Answer from the drawing. Dimensions are ordinates in mm from the lowest x, y and z of the part. A direction names the side the tool comes from. Coordinates: 2 decimals unless noted, no trailing zeros. Loops run counter-clockwise (first coordinate to the right, second up) from the corner with the lowest first, then second, coordinate; pieces in that order, holes last. Notation, with made-up numbers: (53.25, 66.5) - (107.25, 66.5) arc R24 ccw to (107.25, 86.5) - close; hole circle Ø1 at (42, 42.25). An arc over 180 degrees is marked (long way). Use one line per item in the form item = value. Start each with the question number.
1) A cutting plane is placed at A-A (z = 37). Give the vertices of the cut face in (x, y).
2) Each of these flat-tipped pins is pushed along its axis until it touches: P1, Ø20.5, axis at x = 91, y = 65, coming from the +Z side; P2, Ø6, axis at y = 8, z = 78.5, coming from the -X side; P3, Ø1.5, axis at x = 19, y = 46, coming from the -Z side; P4, Ø12.5, axis at x = 66, y = 62, coming from the +Z side. Where does it stop, or does it pass through?
3) A cutting plane is placed at C-C (z = 68). Give the vertices of the cut face in (x, y).
4) Which of the six approach directions +Z, -Z, +X, -X, +Y, -Y give full straight-line access (tool end or side, diameter ignored) to the marked faces 4, 5 and 6?
5) A cutting plane is placed at D-D (x = 66). Give the vertices of the cut face in (y, z).
6) The mould has two halves that part along X. Classify the marked faces 1, 2 and 3: released by +X, released by -X, zero draft, split by the parting line, or undercut.
7) A cutting plane is placed at B-B (y = 59). Give the vertices of the cut face in (x, z).
8) Consider line 1 (X direction, y = 58, z = 42); line 2 (X direction, y = 4, z = 89); line 3 (Y direction, x = 93.5, z = 17.5). Determine where each line is inside the solid, lowest interval first.
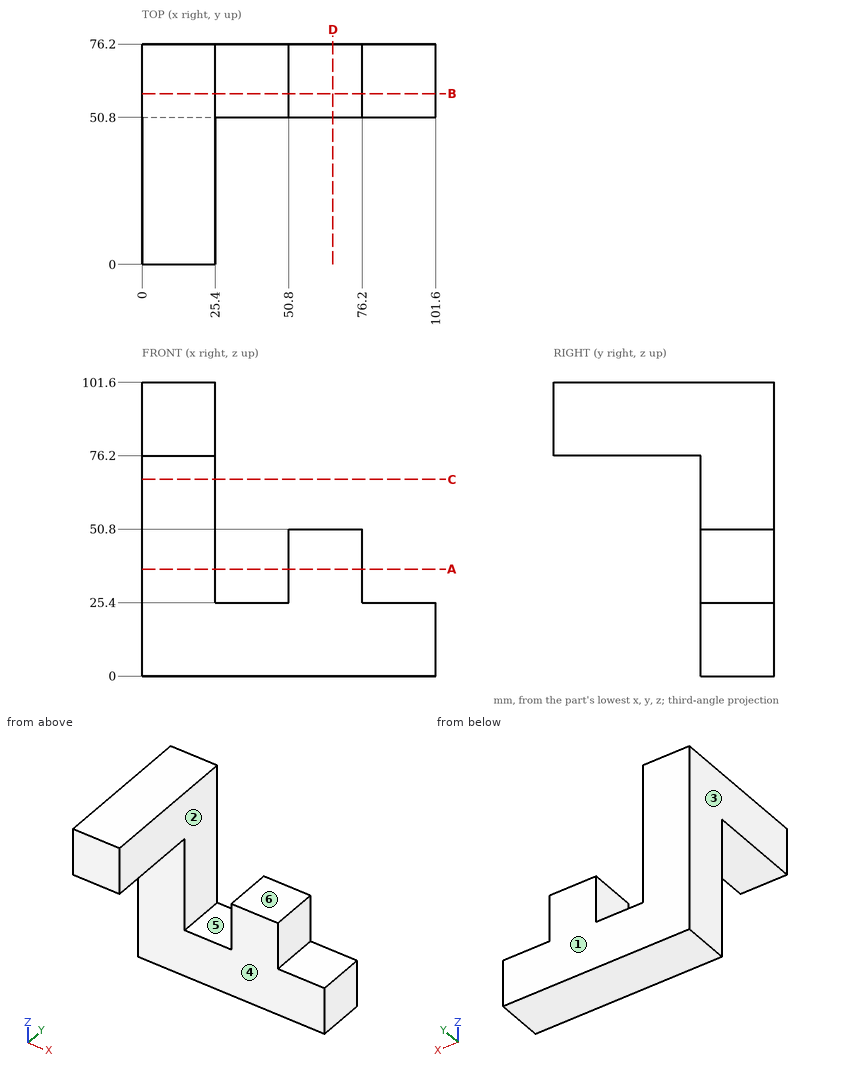
Found:
q1.outline = (0, 50.8) - (25.4, 50.8) - (25.4, 76.2) - (0, 76.2) - close; (50.8, 50.8) - (76.2, 50.8) - (76.2, 76.2) - (50.8, 76.2) - close
q2.P1 = 25.4
q2.P2 = 0
q2.P3 = 76.2
q2.P4 = 50.8
q3.outline = (0, 50.8) - (25.4, 50.8) - (25.4, 76.2) - (0, 76.2) - close
q4.face_4 = -Z, +X, -X, -Y
q4.face_5 = +Z, +Y, -Y
q4.face_6 = +Z, +X, +Y, -Y
q5.outline = (50.8, 0) - (76.2, 0) - (76.2, 50.8) - (50.8, 50.8) - close
q6.face_1 = zero draft
q6.face_2 = undercut
q6.face_3 = released by -X
q7.outline = (0, 0) - (101.6, 0) - (101.6, 25.4) - (76.2, 25.4) - (76.2, 50.8) - (50.8, 50.8) - (50.8, 25.4) - (25.4, 25.4) - (25.4, 101.6) - (0, 101.6) - close
q8.line_1 = 0 to 25.4, 50.8 to 76.2
q8.line_2 = 0 to 25.4
q8.line_3 = 50.8 to 76.2
